Geometry check sheet. Reference: the model listing, model coordinates, mm. A direction names the side the tool comes from. Round coordinates to 2 decimals unless told otherwise and drop trailing zeros. Write each loop counter-clockwise with the first axis right and the second up, starting at its lowest first coordinate (ties: lowest second). Pieces come first, ordered by that corner, then holes. Notation, with made-up numbers: (25.25, -35) - (42.25, -35) arc R26 ccw to (42.25, -9) - close; hole circle Ø9 at (78, 28). An arc over 180 degrees is marked (long way). Return JSON: item names as keys, results as strings.
```python
from build123d import *

# Parameters (mm, degrees)
F1_DEPTH = 10
F2_T     = -2
F3_W     = 12
F3_H     = 8
F4_DEPTH = 2
F5_R     = 2.3
F6_DEPTH = 3
F7_R     = 10
F8_DEPTH = 25


with BuildPart() as f1:
    # F0 (on Front) → F1 (new body)
    with BuildSketch(Plane.XZ):
        with BuildLine():
            Line((-0.003568, 53), (-0.003093, -53))
            ThreePointArc((-0.003093, -53), (53, 0.000237), (-0.003568, 53))
        make_face()
    extrude(amount=F1_DEPTH)

    # F2
    f2_openings = [f1.faces().sort_by_distance(p)[0] for p in [
        (22.492099, -10, 0.000101),
    ]]
    offset(amount=F2_T, openings=f2_openings)

    # F3 (on Front) → F4 (join)
    with BuildSketch(Plane.XZ):
        with Locations((-6, 0)):
            Rectangle(F3_W, F3_H)
    extrude(amount=F4_DEPTH)

    # F5 (on face) → F6 (cut)
    with BuildSketch(Plane(origin=(0, 0, 0), x_dir=(-1, 0, 0), z_dir=(0, 1, 0))):
        with Locations((7.3, 0)):
            Circle(F5_R)
    extrude(amount=-F6_DEPTH, mode=Mode.SUBTRACT)

    # F7 (on face) → F8 (cut)
    with BuildSketch(Plane.XZ.offset(2)):
        with Locations((24.209062, 20.817809)):
            Circle(F7_R)
    extrude(amount=-F8_DEPTH, mode=Mode.SUBTRACT)


solid = f1.part
```
(1) Section check B-B, the plane z = 0. Enter the section's corners in (x, y).
Response values:
{"outline": "(-12, -2) - (-9.6, -2) - (-9.6, 0) - (-12, 0) - close; (-5, -2) - (0, -2) - (0, -10) - (2, -10) - (2, -2) - (51, -2) - (51, -10) - (53, -10) - (53, 0) - (-5, 0) - close"}
(2) Release check for a two-part mould opening along Z. For faces 6 (the face through (-6, -1, 4)), 7 (the face through (21, -2, 1)), 8 (the face through (1, -10, 0)), 9 (the face through (22.041, -1.014, 11.056)) record: pulls with the +Z half, pulls with the -Z half, needs draft (parallel to the pull), parting line crosses it, or undercut.
Response values:
{"face 6": "pulls with the +Z half", "face 7": "undercut", "face 8": "needs draft", "face 9": "undercut"}
(3) Gauge pin test, flat ends, axial feed: pin 1 (1.6 mm diameter, centred on x = -6, y = -1, fed in from +Z); pin 2 (6.5 mm diameter, centred on x = -6, z = 1.5, fed in from -Y); pin 3 (4 mm diameter, centred on x = 6, y = -5, fed in from -Z). Record the tip position at first contact, or that the pin passes through.
Response values:
{"pin 1": "stops at z = 4", "pin 2": "stops at y = -2", "pin 3": "stops at z = -52.85"}
(4) Material ranges on line 1 along Z through (x, y) = (-7.3, -0.6); line 2 along Y through (x, z) = (5, -10.5); line 3 along Z through (x, y) = (43, -4.5), recorded low to high. Write a range as [from, to].
Response values:
{"line 1": "z = [-4, -2.3], [2.3, 4]", "line 2": "y = [-2, 0]", "line 3": "z = [-30.98, -27.42], [27.42, 30.98]"}
(5) Access from +Z, -Z, +X, -X, +Y, -Y to the whole of each face (thin tool, end or side, straight path). Record for faces 1 (the face through (-5, -1, 0)), 2 (the face through (52.987, -4.93, -1.165)), 3 (the face through (-4.8, -2, 0.1)), 4 (the face through (-6, -1, -4)), 5 (the face through (50.99, -5.94, -1.09)).
Response values:
{"face 1": "+Y, -Y", "face 2": "+X, +Y, -Y", "face 3": "+Z, -Z, -X, -Y", "face 4": "-Z, -X, +Y, -Y", "face 5": "-Y"}
(6) Section check C-C, the plane y = -4. Enter the section's corners in (x, z).
Response values:
{"outline": "(0, -53) arc R53 ccw to (0, 53) - close; hole (2, -50.96) arc R51 ccw to (2, 50.96) - close"}
(7) Section check D-D, the plane x = 49. Enter the section's corners in (y, z), plus the area to 3 significant figures.
Response values:
{"outline": "(-10, -20.2) - (0, -20.2) - (0, 20.2) - (-10, 20.2) - (-10, 14.14) - (-2, 14.14) - (-2, -14.14) - (-10, -14.14) - close", "area": "178 mm^2"}
(8) Section check A-A, the plane x = -7.3. Enter the section's corners in (y, z), plus the area to 3 significant figures.
Response values:
{"outline": "(-2, -4) - (0, -4) - (0, -2.3) - (-2, -2.3) - close; (-2, 2.3) - (0, 2.3) - (0, 4) - (-2, 4) - close", "area": "6.80 mm^2"}
